Part print with two shaded views. Sizes in mm from the minimum x, y, z corner. A direction names the side the tool comes from. Round coordinates to 2 decimals unless told otherwise and drop trailing zeros. Loops run counter-clockwise (first coordinate to the right, second up) from the corner with the lowest first, then second, coordinate; pieces in that order, holes last. Notation, with made-up numbers: M -28.75,-4.5 L 30.25,-4.5 A26 ccw 30.25,34.5 Z; hole C -18.5,72 d11. An arc over 180 degrees is marked long. Put each result on its own line as item: value. Start each with the question number.
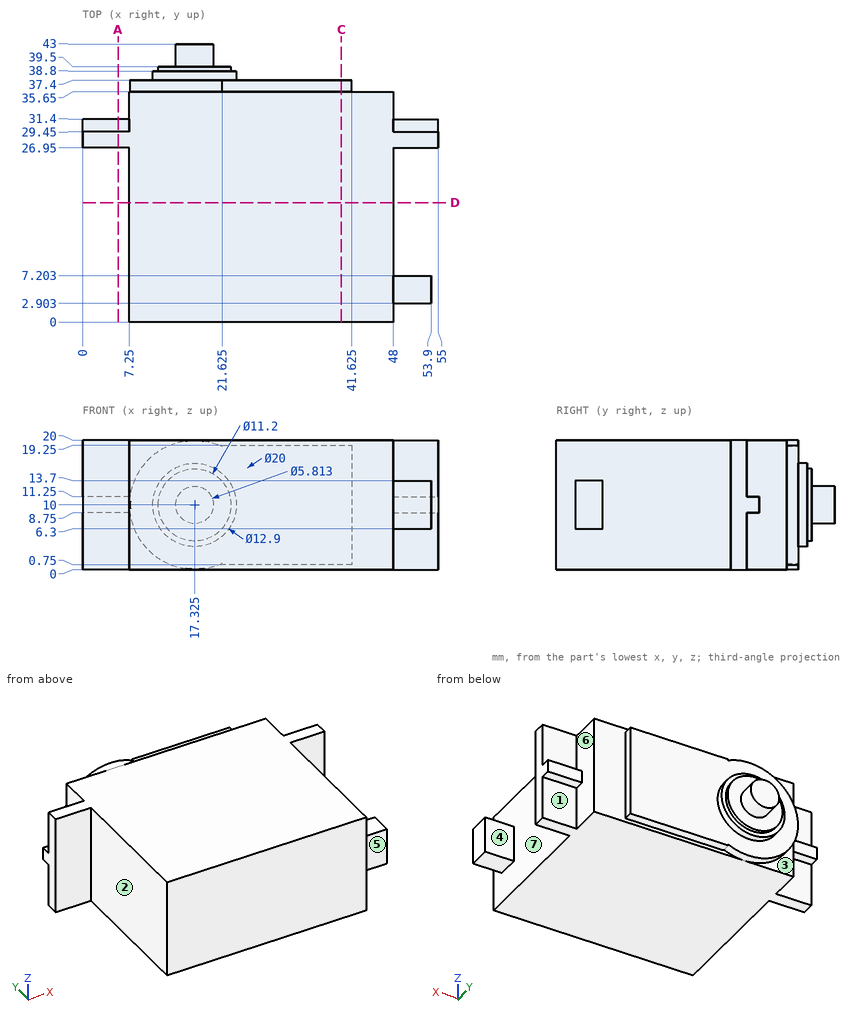
(1) Mould opens along Y. For the marked faces 5, 6 and 7 say: +Y half, -Y half, draft (parallel to the pull), parting line (faces both ways), or undercut.
(2) Flat gauge pins, fed straight in: pin 1 Ø1 at (x, z) = (37, 8) entering from -Y; pin 2 Ø1.2 at (x, z) = (5, 10.5) entering from +Y; pin 3 Ø2 at (x, z) = (3.5, 16.5) entering from +Y; pin 4 Ø3 at (y, z) = (36, 7.5) entering from -X. Where does each tip first touch, or does it go through?
(3) Drill centre lines: line 1 along X through (y, z) = (21, 10.75); line 2 along Y through (x, z) = (35, 18.75); line 3 along Y through (x, z) = (44, 8.5). Where is each one in solid material? Low to high.
(4) Cut at C-C on x = 40. List the corners of the cut face in (y, z), and give its area (3 significant figures).
(5) Cut at D-D on y = 18.5. List the corners of the cut face in (x, z), and give its area (3 significant figures).
(6) Cut at A-A on x = 5.5. List the corners of the cut face in (y, z).
(7) Tool access for the marked faces 1, 2, 3 and 4: list every direction of +Z, -Z, +X, -X, +Y, -Y with a clear straight run to the whole face (end or side of a thin tool).
Taken from the geometry:
1. face 5: -Y half
1. face 6: draft
1. face 7: undercut
2. pin 1: y = 0
2. pin 2: y = 31.4
2. pin 3: y = 29.45
2. pin 4: x = 7.25
3. line 1: 7.25 to 48
3. line 2: 0 to 37.4
3. line 3: 0 to 35.65
4. outline: M 0,0 L 35.65,0 L 35.65,0.75 L 37.4,0.75 L 37.4,19.25 L 35.65,19.25 L 35.65,20 L 0,20 Z
4. area: 745 mm2
5. outline: M 7.25,0 L 48,0 L 48,20 L 7.25,20 Z
5. area: 815 mm2
6. outline: M 26.95,0 L 29.45,0 L 29.45,8.75 L 31.4,8.75 L 31.4,11.25 L 29.45,11.25 L 29.45,20 L 26.95,20 Z
7. face 1: -Z, +X, +Y
7. face 2: +Z, -Z, -X, -Y
7. face 3: -X, +Y
7. face 4: +Z, -Z, +X
